Source: CAD feature listing. Evaluate the final solid. Frame: model axes, mm. Round coordinates to 2 decimals unless told otherwise and drop trailing zeros. Order: outer loops, then holes, each group sorted by start corner. A loop starts at its lowest first (then second) coordinate and runs counter-clockwise, first axis right, second up. Notation, with made-up numbers: M 69.5,27.25 L 97.5,27.25 A10 cw 97.5,36.25 Z; hole C 77.25,11.5 d4. An arc over 180 degrees is marked long. Use one line per item in the form item = value. Start each with the question number.
Q1. Material intervals for probe 1 along X at (y, z) = (12, 8); probe 2 along X at (y, z) = (6.5, 2.5), sorted ascending.
Q2. Pull-direction query (X, two-part tool) for faces 1 (the cylindrical face through (-224.85, 11, 7.1)), 2 (the flat face through (-45, 11, 14)), 3 (the cylindrical face through (149.609, 7.605, 7.098)), 4 (the flat face through (153.143, 10, 7)); classes: pulls with the +X half, pulls with the -X half, needs draft (parallel to the pull), parting line crosses it, or undercut.
Q3. Section A-A (z = 5.25). Return the cut outline in (x, y), plus the area to 3 significant figures.
Q4. Contact query for a flat-ended pin moving along its axis: pin 1 (10 mm diameter, centred on x = -46, y = 9, fed in from -Z). Output: stop coordinate, or through.
from build123d import *

# Parameters (mm, degrees)
SKETCH1_W           = 391
SKETCH1_H           = 32
BOSS_EXTRUDE1_DEPTH = 14
SKETCH2_R           = 7
CUT_EXTRUDE1_DEPTH  = 240.714328282
SKETCH3_R           = 7
CUT_EXTRUDE2_DEPTH  = 240.714328282


with BuildPart() as part:
    # Sketch1 → Boss-Extrude1 (new body)
    with BuildSketch(Plane.XY):
        with Locations((-42.357142857, 10.285714286)):
            Rectangle(SKETCH1_W, SKETCH1_H)
    extrude(amount=BOSS_EXTRUDE1_DEPTH)

    # Sketch2 → Cut-Extrude1 (cut, through all)
    with BuildSketch(Plane.XY.offset(14)):
        with Locations((-217.857142857, 10.691731498)):
            Circle(SKETCH2_R)
    extrude(amount=-CUT_EXTRUDE1_DEPTH, mode=Mode.SUBTRACT)

    # Sketch3 → Cut-Extrude2 (cut, through all)
    with BuildSketch(Plane.XY.offset(14)):
        with Locations((143.142857143, 10.285714286)):
            Circle(SKETCH3_R)
    extrude(amount=-CUT_EXTRUDE2_DEPTH, mode=Mode.SUBTRACT)


solid = part.part
Results list:
q1.probe_1 = -237.86 to -224.73, -210.98 to 136.36, 149.93 to 153.14
q1.probe_2 = -237.86 to -223.46, -212.25 to 137.25, 149.03 to 153.14
q2.face_1 = undercut
q2.face_2 = needs draft
q2.face_3 = undercut
q2.face_4 = pulls with the +X half
q3.outline = M -237.86,-5.71 L 153.14,-5.71 L 153.14,26.29 L -237.86,26.29 Z; hole C -217.86,10.69 d14; hole C 143.14,10.29 d14
q3.area = 12,200 mm2
q4.pin_1 = 0
